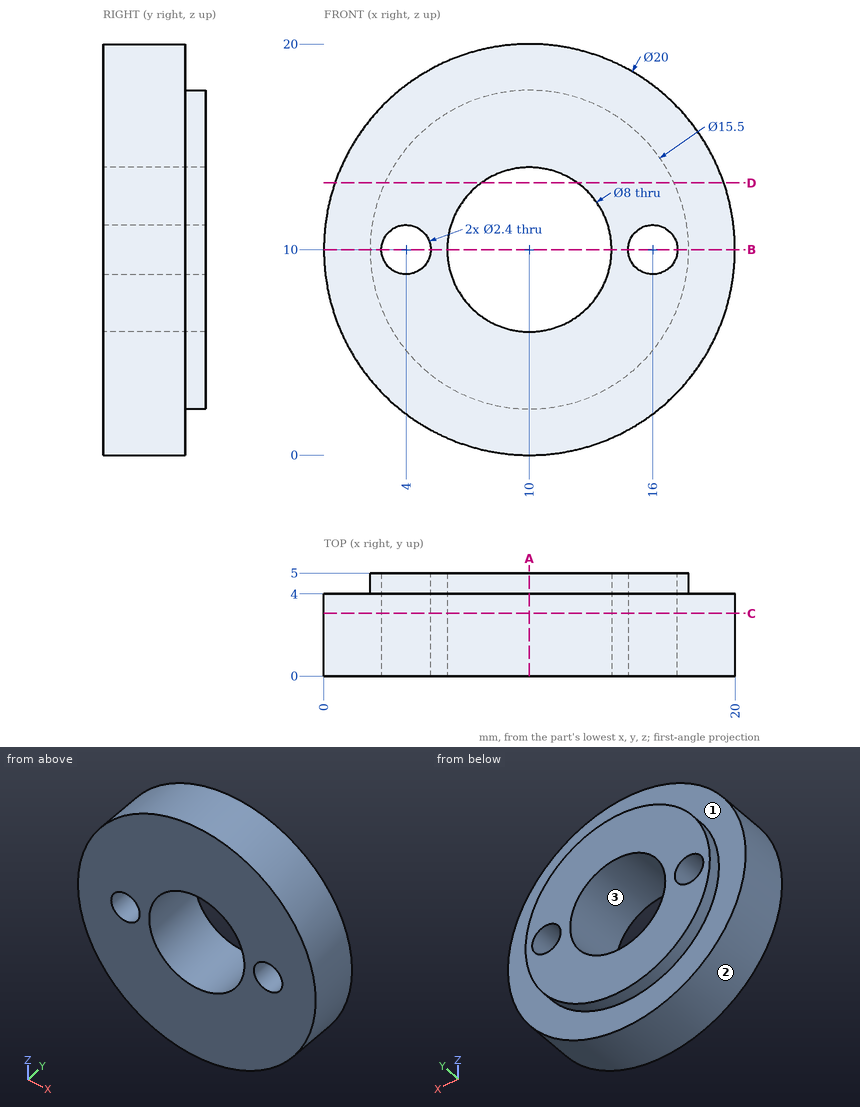
Study the drawing (mm; zero at the part's minimum x, y, z) and answer. Round coordinates to 2 decimals unless told otherwise and drop trailing zeros. Write each loop counter-clockwise with the first axis right and the second up, starting at its lowest first coordinate (ties: lowest second). Pieces come first, ordered by that corner, then holes. Notation, with made-up numbers: (-27.75, 36) - (26.25, 36) arc R35 ccw to (26.25, 72) - close; hole circle Ø8 at (89, 43). An arc over 180 degrees is marked (long way). Use CSV: the item, a comma, the result in double quotes.
Q1. Each of these flat-tipped pins is pushed along its axis until it touches: pin 1 Ø1.5 at (y, z) = (4.5, 5) entering from +X; pin 2 Ø1 at (x, y) = (2.5, 2) entering from -Z; pin 3 Ø2 at (y, z) = (2, 8.5) entering from +X. Where does it stop, or does it pass through?
Values:
pin 1,"stops at x = 18.96"
pin 2,"stops at z = 2.86"
pin 3,"stops at x = 19.99"
Q2. Find section B-B, the plane z = 10. Write down the section's boundary in (x, y), then the cut area to 3 significant figures.
Values:
outline,"(0, 0) - (2.8, 0) - (2.8, 5) - (2.25, 5) - (2.25, 4) - (0, 4) - close; (5.2, 0) - (6, 0) - (6, 5) - (5.2, 5) - close; (14, 0) - (14.8, 0) - (14.8, 5) - (14, 5) - close; (17.2, 0) - (20, 0) - (20, 4) - (17.75, 4) - (17.75, 5) - (17.2, 5) - close"
area,"31.5 mm²"
Q3. Find section D-D, the plane z = 13.25. Write down the section's boundary in (x, y).
Values:
outline,"(0.54, 0) - (7.67, 0) - (7.67, 5) - (2.96, 5) - (2.96, 4) - (0.54, 4) - close; (12.33, 0) - (19.46, 0) - (19.46, 4) - (17.04, 4) - (17.04, 5) - (12.33, 5) - close"
Q4. Find section C-C, the plane y = 3.05. Write down the section's boundary in (x, z), then the cut area to 3 significant figures.
Values:
outline,"circle Ø20 at (10, 10); hole circle Ø2.4 at (4, 10); hole circle Ø8 at (10, 10); hole circle Ø2.4 at (16, 10)"
area,"255 mm²"
Q5. Straight lines are drawn through the part: line 1 along Z through (x, y) = (10, 1); line 2 along Y through (x, z) = (11.5, 1.25); line 3 along Z through (x, y) = (11, 4.3). For each, find the intervals that lie inside material, in ascending order.
Values:
line 1,"z = 0 to 6, 14 to 20"
line 2,"y = 0 to 4"
line 3,"z = 2.31 to 6.13, 13.87 to 17.69"
Q6. Determine the mould class of the marked faces 1, 2 and 3 for opening direction Z: +Z half, -Z half, draft (parallel to the pull), parting line (faces both ways), or undercut.
Values:
face 1,"draft"
face 2,"parting line"
face 3,"undercut"
Q7. Find section A-A, the plane x = 10. Write down the section's boundary in (y, z).
Values:
outline,"(0, 0) - (4, 0) - (4, 2.25) - (5, 2.25) - (5, 6) - (0, 6) - close; (0, 14) - (5, 14) - (5, 17.75) - (4, 17.75) - (4, 20) - (0, 20) - close"
